from build123d import *

# Parameters (mm, degrees)
SKETCH1_R           = 1.5875
BOSS_EXTRUDE1_DEPTH = 1
SKETCH2_R           = 1.5875
BOSS_EXTRUDE2_DEPTH = 12.7


with BuildPart() as part:
    # Sketch1 → Boss-Extrude1 (new body)
    with BuildSketch(Plane(origin=(0, 0, 0), x_dir=(1, 0, 0), z_dir=(0, 1, 0))):
        Polygon((25.4, 9.525), (25.4, 1.5875), (19.05, 1.5875), (19.05, 0), (6.35, 0), (6.35, 1.5875), (0, 1.5875), (0, 9.525), align=None)
        with Locations(Location((4.7625, 4.7625, 0), (0, 0, 270))):
            Circle(SKETCH1_R, mode=Mode.SUBTRACT)
        with Locations(Location((20.6375, 4.7625, 0), (0, 0, 90))):
            Circle(SKETCH1_R, mode=Mode.SUBTRACT)
    extrude(amount=BOSS_EXTRUDE1_DEPTH)

    # Sketch2 → Boss-Extrude2 (add)
    with BuildSketch(Plane.ZY.offset(-6.35)):
        with Locations((0, 1.5875)):
            Circle(SKETCH2_R)
    extrude(amount=-BOSS_EXTRUDE2_DEPTH)


solid = part.part
Could you check a few things on this model? Use its own coordinates, in mm. A direction names the side the tool comes from. Give positions to 0.01 mm unless a question says otherwise; leave off trailing zeros. Order: outer loops, then holes, each group sorted by start corner. A loop starts at its lowest first (then second) coordinate and runs counter-clockwise, first axis right, second up. Notation, with made-up numbers: (0, -2.5) - (58, -2.5) arc R24 ccw to (58, 14.5) - close; hole circle Ø5 at (-34, -10.5). An arc over 180 degrees is marked (long way). Return JSON: item names as keys, results as strings. Group by question number.
Q1. Suppose I cut it at D-D, the plane y = 1.65. Please give me the cut outline in (x, z), and give its area (3 significant figures).
Q2. Suppose I cut it at A-A, the plane y = 0.3. State how many separate pieces and enclosed holes the cut face has, and give its area (3 significant figures).
Q3. Suppose I cut it at C-C, the plane x = 2.5. Please give me the cut outline in (y, z) (1 decimal), and give its area (3 significant figures).
Q4. Suppose I cut it at B-B, the plane z = -5.75. Please give me the cut outline in (x, y), and give its area (3 significant figures).
Q5. Will these pins go through, and if not, where does the flat tip stop? pin 1 Ø4 at (x, z) = (18, -8.5) entering from -Y; pin 2 Ø6.5 at (x, z) = (8, -4) entering from +Y; pin 3 Ø0.8 at (x, y) = (21.5, 0.5) entering from +Z; pin 4 Ø1 at (y, z) = (1, 0) entering from -X.
Q6. Thinking about a two-plate mould opening in Z: for faces 1 (the face through (19.05, 2, 0)), 2 (the face through (3.2, 0.5, -1.588)), 3 (the face through (5.84, 0.49, -5.93)), 4 (the face through (20.161, 0.493, -6.277)), which applies, pulls with the +Z half, pulls with the -Z half, needs draft (parallel to the pull), parting line crosses it, or undercut?
Q7. Which directions (+Z, -Z, +X, -X, +Y, -Y) give clear straight access to the entire face, cutting with the end or side of a thin tool? Please do faces 5 (the face through (6.35, 2, 0)), 6 (the face through (12.5, 0.5, -9.525)), 7 (the face through (22.3, 0.5, -1.588)).
Q8. Please list where these lines run through material, in increasing order: line 1 along Y through (x, z) = (14, -4.75); line 2 along X through (y, z) = (0.2, -5.25); line 3 along Z through (x, y) = (4.75, 0.75) (1 decimal). Write a range as [from, to].
Resolved:
{
 "1": {"outline": "(6.35, -1.59) - (19.05, -1.59) - (19.05, 1.59) - (6.35, 1.59) - close", "area": "40.3 mm2"},
 "2": {"separate pieces": "1", "enclosed holes": "2", "area": "218 mm2"},
 "3": {"outline": "(0, -9.5) - (1, -9.5) - (1, -1.6) - (0, -1.6) - close", "area": "7.94 mm2"},
 "4": {"outline": "(0, 0) - (3.52, 0) - (3.52, 1) - (0, 1) - close; (6.01, 0) - (19.39, 0) - (19.39, 1) - (6.01, 1) - close; (21.88, 0) - (25.4, 0) - (25.4, 1) - (21.88, 1) - close", "area": "20.4 mm2"},
 "5": {"pin 1": "stops at y = 0", "pin 2": "stops at y = 2.99", "pin 3": "stops at z = -1.59", "pin 4": "stops at x = 6.35"},
 "6": {"face 1": "needs draft", "face 2": "pulls with the +Z half", "face 3": "undercut", "face 4": "undercut"},
 "7": {"face 5": "+Z, -X, +Y, -Y", "face 6": "-Z, +X, -X, +Y, -Y", "face 7": "+Z, +X, +Y, -Y"},
 "8": {"line 1": "y = [0, 1]", "line 2": "x = [0, 3.25], [6.27, 19.13], [22.15, 25.4]", "line 3": "z = [-9.5, -6.3], [-3.2, -1.6]"}
}
